Can you work these out from the model? Positions are in its coordinate system, mm. Face numbers are marked on the shaded views. A direction names the side the tool comes from. Give positions to 0.01 mm unless a question says otherwise; leave off trailing zeros. Order: outer loops, then holes, each group sorted by start corner. A loop starts at its lowest first (then second) coordinate and runs counter-clockwise, first axis right, second up. Notation, with made-up numbers: (73.25, -20.5) - (123.25, -20.5) arc R9 ccw to (123.25, -4.5) - close; hole circle Ø6 at (80, 14). An arc over 180 degrees is marked (long way). Answer as a JSON object with one key per item and string values.
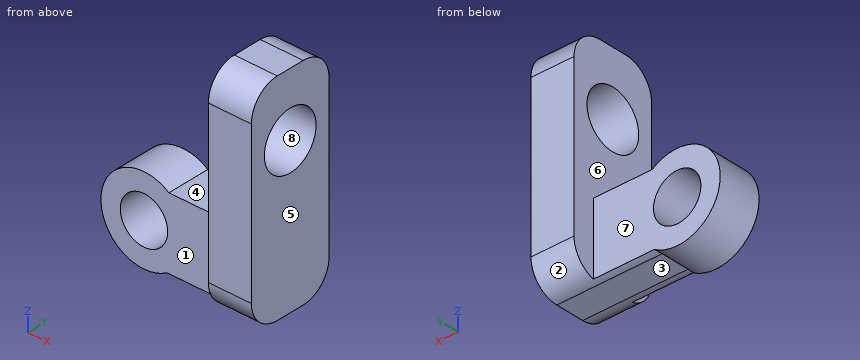
```python
from build123d import *

# Parameters (mm, degrees)
F0_R          = 3
F0_R_2        = 1.65
F1_DEPTH      = 1.5
F1_DEPTH_BACK = 1.5
F3_DEPTH      = 1.5
F3_DEPTH_BACK = 1.5
F4_W          = 3
F4_H          = 15.04355
F5_DEPTH      = 3
F5_DEPTH_BACK = 3
F6_R          = 2
F7_DEPTH      = 25
F8_R          = 2


with BuildPart() as f1:
    # F0 (on Front) → F1 (new body, two sides)
    with BuildSketch(Plane.XZ) as f1_sk:
        Circle(F0_R)
        Circle(F0_R_2, mode=Mode.SUBTRACT)
    extrude(amount=F1_DEPTH)
    extrude(f1_sk.sketch, amount=-F1_DEPTH_BACK)

    # F2 (on Front) → F3 (join, two sides)
    with BuildSketch(Plane.XZ) as f3_sk:
        with BuildLine():
            Line((7.740623, 2.443406), (1.740623, 2.443406))
            ThreePointArc((1.740623, 2.443406), (2.666633, 1.374433), (3, 0))
            ThreePointArc((3, 0), (2.59704, -1.501793), (1.496413, -2.600144))
            Line((1.496413, -2.600144), (7.740623, -2.600144))
            Line((7.740623, -2.600144), (7.740623, 2.443406))
        make_face()
    extrude(amount=F3_DEPTH)
    extrude(f3_sk.sketch, amount=-F3_DEPTH_BACK)

    # F4 (on Front) → F5 (join, two sides)
    with BuildSketch(Plane.XZ) as f5_sk:
        with Locations((7.336591, 4.921631)):
            Rectangle(F4_W, F4_H)
    extrude(amount=F5_DEPTH)
    extrude(f5_sk.sketch, amount=-F5_DEPTH_BACK)

    # F6 (on face) → F7 (cut)
    with BuildSketch(Plane(origin=(5.836591, 0, 0), x_dir=(0, -1, 0), z_dir=(-1, 0, 0))):
        with Locations((0, 8)):
            Circle(F6_R)
    extrude(amount=-F7_DEPTH, mode=Mode.SUBTRACT)

    # F8
    f8_edges = [f1.edges().sort_by_distance(p)[0] for p in [
        (7.336591, -3, 12.443406),
        (7.336591, 3, 12.443406),
        (7.336591, -3, -2.600144),
        (7.336591, 3, -2.600144),
    ]]
    fillet(f8_edges, radius=F8_R)


solid = f1.part
```
Q1. I'm going to push flat-ended pins straight in: pin 1 Ø1.6 at (x, y) = (6.5, 0.5) entering from -Z; pin 2 Ø5 at (x, z) = (-0.5, 1) entering from -Y; pin 3 Ø0.9 at (x, y) = (4.5, 0) entering from +Z; pin 4 Ø4 at (x, z) = (3, 8.5) entering from +Y. Where does each tip first touch, or does it pass through?
Recorded:
{"pin 1": "stops at z = -2.6", "pin 2": "stops at y = -1.5", "pin 3": "stops at z = 2.44", "pin 4": "passes through"}
Q2. Which directions (+Z, -Z, +X, -X, +Y, -Y) give clear straight access to the entire face, cutting with the end or side of a thin tool? Please do the marked faces 1, 2, 3, 4 and 5.
Recorded:
{"face 1": "+Z, -Z, -X, -Y", "face 2": "-Z, +X, +Y", "face 3": "-Z, +X, +Y, -Y", "face 4": "+Z, +Y, -Y", "face 5": "+Z, -Z, +X, +Y, -Y"}
Q3. If we section it at A-A, the plane z = 0: Please give me the cut outline in (x, y), then the cut area to 3 significant figures.
Recorded:
{"outline": "(-3, -1.5) - (-1.65, -1.5) - (-1.65, 1.5) - (-3, 1.5) - close; (1.65, -1.5) - (5.84, -1.5) - (5.84, -3) - (8.84, -3) - (8.84, 3) - (5.84, 3) - (5.84, 1.5) - (1.65, 1.5) - close", "area": "34.6 mm^2"}
Q4. If we section it at B-B, the plane y = 0: Please give me the cut outline in (x, z).
Recorded:
{"outline": "(1.5, -2.6) - (8.84, -2.6) - (8.84, 6) - (5.84, 6) - (5.84, 2.44) - (1.74, 2.44) arc R3 ccw (long way) to start; (5.84, 10) - (8.84, 10) - (8.84, 12.44) - (5.84, 12.44) - close; hole circle Ø3.3 at (0, 0)"}
Q5. If we section it at D-D, the plane x = 6: Please give me the cut outline in (y, z), then the cut area to 3 significant figures.
Recorded:
{"outline": "(-3, -0.6) arc R2 ccw to (-1, -2.6) - (1, -2.6) arc R2 ccw to (3, -0.6) - (3, 10.44) arc R2 ccw to (1, 12.44) - (-1, 12.44) arc R2 ccw to (-3, 10.44) - close; hole circle Ø4 at (0, 8)", "area": "74.3 mm^2"}
Q6. I need wall thicknesses on L1, parallel to Z at x = 0, y = 0.2; L2, parallel to Z at x = 6.85, y = 0; L3, parallel to Z at x = 5, y = -1. Which ranges of each line are inside material? Lowest first, please.
Recorded:
{"L1": "z = -3 to -1.65, 1.65 to 3", "L2": "z = -2.6 to 6, 10 to 12.44", "L3": "z = -2.6 to 2.44"}
Q7. If we section it at C-C, the plane x = 0: Please give me the cut outline in (y, z), then the cut area to 3 significant figures.
Recorded:
{"outline": "(-1.5, -3) - (1.5, -3) - (1.5, -1.65) - (-1.5, -1.65) - close; (-1.5, 1.65) - (1.5, 1.65) - (1.5, 3) - (-1.5, 3) - close", "area": "8.10 mm^2"}
Q8. We'd pull the mould along Y, two halves only. Please class the marked faces 6, 7 and 8: released by +Y, released by -Y, zero draft, split by the parting line, or undercut.
Recorded:
{"face 6": "zero draft", "face 7": "released by +Y", "face 8": "undercut"}
